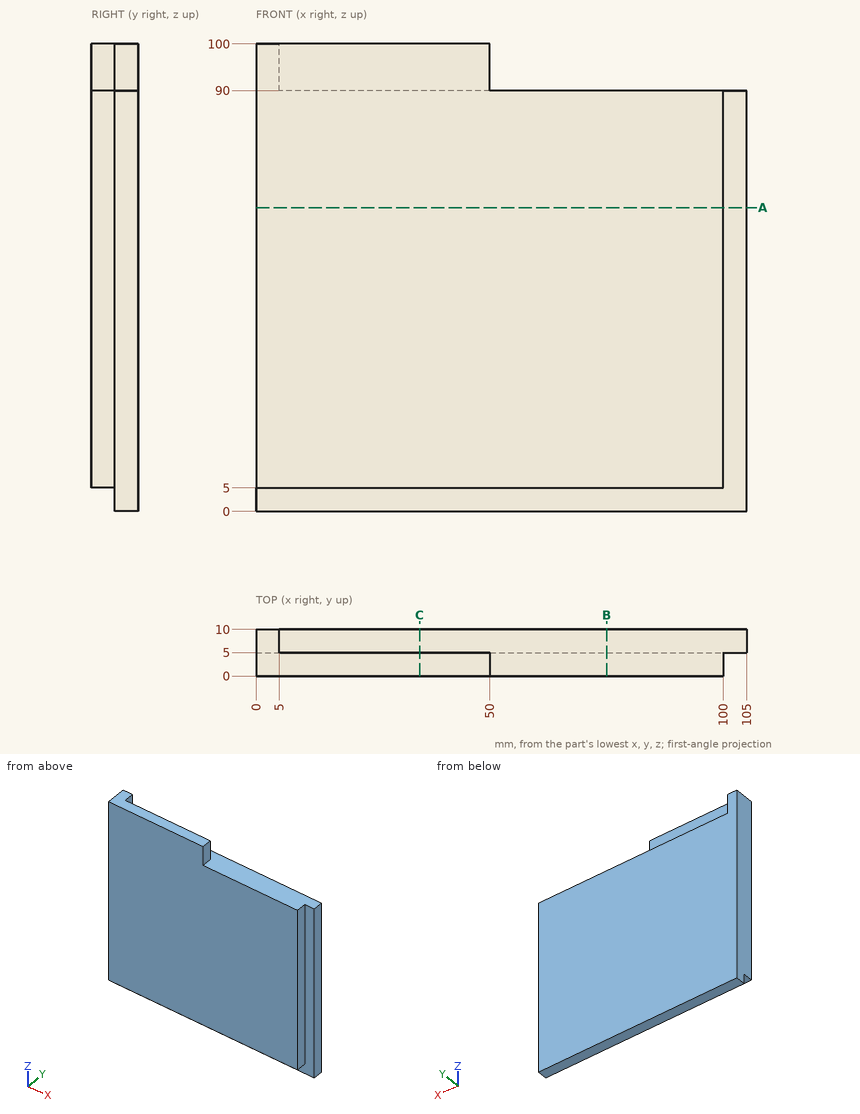
Geometry check sheet. Reference: drawing and pictorial views, mm from the part's lowest x, y, z. Round coordinates to 2 decimals unless told otherwise and drop trailing zeros. Order: outer loops, then holes, each group sorted by start corner. A loop starts at its lowest first (then second) coordinate and runs counter-clockwise, first axis right, second up. Notation, with made-up numbers: M 36,34 L 85,34 A12 cw 85,49 Z; hole C 79,7.25 d8. An arc over 180 degrees is marked long. Answer in a Markdown table with one row per item.
(1) Sectioned sample at A-A, the plane z = 65. Record the cut outline in (x, y).
Responses:
| item | result |
|---|---|
| outline | M 0,0 L 100,0 L 100,5 L 105,5 L 105,10 L 0,10 Z |
(2) Go/stop test with flat-tipped pins: P1, Ø3, axis at x = 38.5, z = 95, coming from the +Y side; P2, Ø3, axis at x = 60, y = 5.5, coming from the +Z side; P3, Ø5.5, axis at y = 3.5, z = 93, coming from the +X side; P4, Ø4, axis at y = 6, z = 14.5, coming from the -X side. Record where each tip stops, or that it passes through.
Responses:
| item | result |
|---|---|
| P1 | stops at y = 5 |
| P2 | stops at z = 90 |
| P3 | stops at x = 50 |
| P4 | stops at x = 0 |
(3) Sectioned sample at C-C, the plane x = 35. Record the cut outline in (y, z), and give its area (3 significant figures).
Responses:
| item | result |
|---|---|
| outline | M 0,5 L 5,5 L 5,0 L 10,0 L 10,90 L 5,90 L 5,100 L 0,100 Z |
| area | 925 mm² |
(4) Scan lines: probe 1 along Z at (x, y) = (6, 8.75); probe 2 along X at (y, z) = (3, 35); probe 3 along Y at (x, z) = (101.5, 51). Record each from-to range of solid material in increasing order. Write a range as from..to.
Responses:
| item | result |
|---|---|
| probe 1 | z = 0..90 |
| probe 2 | x = 0..100 |
| probe 3 | y = 5..10 |
(5) Sectioned sample at B-B, the plane x = 75. Record the cut outline in (y, z).
Responses:
| item | result |
|---|---|
| outline | M 0,5 L 5,5 L 5,0 L 10,0 L 10,90 L 0,90 Z |
